```python
from build123d import *

# Parameters (mm, degrees)
BOSS_EXTRUDE1_DEPTH      = 63.5
BOSS_EXTRUDE1_DEPTH_BACK = 63.5


with BuildPart() as part:
    # Sketch1 → Boss-Extrude1 (new body, two sides)
    with BuildSketch(Plane.XY) as boss_extrude1_sk:
        with BuildLine():
            ThreePointArc((3.175, 0), (-1.419903166, 2.839806331), (-1.905, -2.54))
            Line((-1.905, -2.54), (1.905, -2.54))
            ThreePointArc((1.905, -2.54), (2.839806331, -1.419903166), (3.175, 0))
        make_face()
    extrude(amount=BOSS_EXTRUDE1_DEPTH)
    extrude(boss_extrude1_sk.sketch, amount=-BOSS_EXTRUDE1_DEPTH_BACK)


solid = part.part
```
Can you work these out from the model? Positions are in its coordinate system, mm. Round coordinates to 2 decimals unless told otherwise and drop trailing zeros. Loops run counter-clockwise (first coordinate to the right, second up) from the corner with the lowest first, then second, coordinate; pieces in that order, holes last. Notation, with made-up numbers: M 65.25,47 L 70.25,47 A18 ccw 70.25,75 Z; hole C 3.5,-13 d1. An arc over 180 degrees is marked long. Answer in a Markdown table with one row per item.
1. If we section it at B-B, the plane y = 1.5: Please give me the cut outline in (x, z), plus the area to 3 significant figures.
Established:
| item | result |
|---|---|
| outline | M -2.8,-63.5 L 2.8,-63.5 L 2.8,63.5 L -2.8,63.5 Z |
| area | 711 mm² |
2. Please list where these lines run through material, in increasing order: line 1 (X direction, y = 0.1, z = 54.5); line 2 (Y direction, x = 0.25, z = -49.5); line 3 (Y direction, x = -1.75, z = -46.5). Write a range as from..to.
Established:
| item | result |
|---|---|
| line 1 | -3.17..3.17 |
| line 2 | -2.54..3.17 |
| line 3 | -2.54..2.65 |
3. If we section it at A-A, the plane z = 39.5: Please give me the cut outline in (x, y) (3 decimals).
Established:
| item | result |
|---|---|
| outline | M -1.905,-2.54 L 1.905,-2.54 A3.175 ccw long Z |
4. I'm going to push a flat-ended pin straight in: pin 1 Ø1 at (y, z) = (-0.5, -32) entering from +X (3 decimals). Where does the tip first touch, or does it pass through?
Established:
| item | result |
|---|---|
| pin 1 | x = 3.175 |
